Here's how the part is built. I have some questions about the finished solid (model axes, mm). A direction names the side the tool comes from. Coordinates: 2 decimals unless noted, no trailing zeros. Order: outer loops, then holes, each group sorted by start corner. A loop starts at its lowest first (then second) coordinate and runs counter-clockwise, first axis right, second up. Notation, with made-up numbers: (79, 85.5) - (118, 85.5) arc R34 ccw to (118, 121.5) - close; hole circle Ø3 at (72, -18.5). An arc over 180 degrees is marked (long way). Answer in a Markdown table with one row per item. Add a question column.
Item 1: I want a section at B-B (x = -25). Please give me the cut outline in (y, z).
Item 2: Thinking about a two-plate mould opening in Y: for faces 4 (the flat face through (-25, 9, 4)), 5 (the flat face through (-25, 0, 2)), 6 (the cylindrical face through (-22.854, 5.676, 5.356)), 7 (the flat face through (-15.28, 15.73, 1.97)), which applies, +Y half, -Y half, draft (parallel to the pull), parting line (faces both ways), or undercut?
Item 3: I want a section at C-C (y = 19.75). Please give me the cut outline in (x, z), plus the area to 3 significant figures.
Item 4: I want a section at D-D (z = -1.5). Please give me the cut outline in (x, y), plus the area to 3 significant figures.
Item 5: I want a section at A-A (z = 2). Please give me the cut outline in (x, y).
Item 6: On a 3-axis mill with a long thin cutter (end or side, diameter ignored), from which of +Z, -Z, +X, -X, +Y, -Y can I reach the whole of each face in a straight line? I mean faces 1 (the cylindrical face through (-22.854, 5.676, -1.356)), 2 (the flat face through (-9, 5, 2)), 3 (the flat face through (-41, 5, 2)). Say none if no direction works.
Item 7: Will these pins go through, and if not, where does the flat tip stop? pin 1 Ø2 at (y, z) = (7, 2) entering from -X; pin 2 Ø3 at (x, z) = (-7, 1.5) entering from +Y; pin 3 Ø11 at (x, y) = (-28.5, 8) entering from -Z; pin 4 Ø8 at (x, y) = (-32.5, 6.5) entering from +Z.
Item 8: If I drill on line 1 along Z through (x, y) = (-18.5, 13); line 2 along X through (y, z) = (6, 5); line 3 along X through (y, z) = (15.25, 1), over which ranges is the centre line in solid material (lowest first)? Write a range as from..to.
```python
from build123d import *

# Parameters (mm, degrees)
BOSS_EXTRUDE1_DEPTH      = 4
SKETCH2_R                = 2.25
BOSS_EXTRUDE2_DEPTH      = 3
BOSS_EXTRUDE2_DEPTH_BACK = 7
FILLET1_R                = 0.25


with BuildPart() as part:
    # Sketch1 → Boss-Extrude1 (new body)
    with BuildSketch(Plane.XY):
        Polygon((-50, 0), (0, 0), (0, 5), (-17.5, 5), (-17.5, 9.636351612), (-13, 22), (-37, 22), (-32.5, 9.636351612), (-32.5, 5), (-50, 5), align=None)
    extrude(amount=BOSS_EXTRUDE1_DEPTH)

    # Sketch2 → Boss-Extrude2 (add, two sides)
    with BuildSketch(Plane.XY.offset(4)) as boss_extrude2_sk:
        with Locations((-25, 5)):
            Circle(SKETCH2_R)
    extrude(amount=BOSS_EXTRUDE2_DEPTH)
    extrude(boss_extrude2_sk.sketch, amount=-BOSS_EXTRUDE2_DEPTH_BACK)

    # Fillet1
    fillet1_edges = [part.edges().sort_by_distance(p)[0] for p in [
        (-27.25, 5, -3),
        (-27.25, 5, 7),
    ]]
    fillet(fillet1_edges, radius=FILLET1_R)


solid = part.part
```
Values follow:
| question | item | result |
|---|---|---|
| 1 | outline | (0, 0) - (2.75, 0) - (2.75, -2.75) arc R0.25 ccw to (3, -3) - (7, -3) arc R0.25 ccw to (7.25, -2.75) - (7.25, 0) - (22, 0) - (22, 4) - (7.25, 4) - (7.25, 6.75) arc R0.25 ccw to (7, 7) - (3, 7) arc R0.25 ccw to (2.75, 6.75) - (2.75, 4) - (0, 4) - close |
| 2 | face 4 | draft |
| 2 | face 5 | -Y half |
| 2 | face 6 | parting line |
| 2 | face 7 | undercut |
| 3 | outline | (-36.18, 0) - (-13.82, 0) - (-13.82, 4) - (-36.18, 4) - close |
| 3 | area | 89.4 mm^2 |
| 4 | outline | circle Ø4.5 at (-25, 5) |
| 4 | area | 15.9 mm^2 |
| 5 | outline | (-50, 0) - (0, 0) - (0, 5) - (-17.5, 5) - (-17.5, 9.64) - (-13, 22) - (-37, 22) - (-32.5, 9.64) - (-32.5, 5) - (-50, 5) - close |
| 6 | face 1 | -Z |
| 6 | face 2 | +Z, -Z, +X |
| 6 | face 3 | +Z, -Z, -X |
| 7 | pin 1 | stops at x = -32.5 |
| 7 | pin 2 | stops at y = 5 |
| 7 | pin 3 | stops at z = -3 |
| 7 | pin 4 | stops at z = 4 |
| 8 | line 1 | z = 0..4 |
| 8 | line 2 | x = -27.02..-22.98 |
| 8 | line 3 | x = -34.54..-15.46 |
